from build123d import *

# Parameters (mm, degrees)
SKETCH1_W                                           = 35
SKETCH1_H                                           = 280
EXTRUDE1_DEPTH                                      = 16
EXTRUDE2_REACH                                      = 282
SKETCH2_W                                           = 15.5
SKETCH2_H                                           = 2.5
M4_TAPPED_HOLE1_D                                   = 3.3
M6_TAPPED_HOLE1_D                                   = 5
CBORE_FOR_M6_HEX_SOCKET_HEAD_CAP_SCREW1_D           = 6.6
CBORE_FOR_M6_HEX_SOCKET_HEAD_CAP_SCREW1_DEPTH       = 29
CBORE_FOR_M6_HEX_SOCKET_HEAD_CAP_SCREW1_CBORE_D     = 11
CBORE_FOR_M6_HEX_SOCKET_HEAD_CAP_SCREW1_CBORE_DEPTH = 6.4
CBORE_FOR_M6_HEX_SOCKET_HEAD_CAP_SCREW1_TIP         = 1.982840043


with BuildPart() as part:
    # Sketch1 → Extrude1 (new body)
    with BuildSketch(Plane.XY):
        Rectangle(SKETCH1_W, SKETCH1_H)
    extrude(amount=EXTRUDE1_DEPTH)

    # Sketch2 → Extrude2 (cut, up to next)
    with BuildSketch(Plane.XZ.offset(140), mode=Mode.PRIVATE) as extrude2_sk1:
        with Locations((-9.75, 14.75)):
            Rectangle(SKETCH2_W, SKETCH2_H)
    extrude2_tool1 = extrude(extrude2_sk1.sketch, amount=-EXTRUDE2_REACH, mode=Mode.PRIVATE) & part.part
    add(extrude2_tool1.solids().sort_by_distance((-9.75, -140, 14.75))[0], mode=Mode.SUBTRACT)

    # M4 Tapped Hole1 (through all)
    with Locations(Plane.XY.offset(13.5)):
        with Locations((-9.5, -120), (-9.5, -60), (-9.5, 0), (-9.5, 60), (-9.5, 120)):
            Hole(M4_TAPPED_HOLE1_D / 2)

    # M6 Tapped Hole1 (through all)
    with Locations(Plane(origin=(0, -140, 0), x_dir=(-1, 0, 0), z_dir=(0, -1, 0))):
        with Locations((-5.5, -7)):
            Hole(M6_TAPPED_HOLE1_D / 2)

    # CBORE for M6 Hex Socket Head Cap Screw1
    with Locations(Plane.XY.offset(16)):
        with Locations((0, 125), (0, 70), (0, 0), (0, -70), (0, -125)):
            CounterBoreHole(CBORE_FOR_M6_HEX_SOCKET_HEAD_CAP_SCREW1_D / 2, CBORE_FOR_M6_HEX_SOCKET_HEAD_CAP_SCREW1_CBORE_D / 2, CBORE_FOR_M6_HEX_SOCKET_HEAD_CAP_SCREW1_CBORE_DEPTH, depth=CBORE_FOR_M6_HEX_SOCKET_HEAD_CAP_SCREW1_DEPTH)
            with Locations((0, 0, -(CBORE_FOR_M6_HEX_SOCKET_HEAD_CAP_SCREW1_DEPTH + CBORE_FOR_M6_HEX_SOCKET_HEAD_CAP_SCREW1_TIP / 2))):  # 118° drill point
                Cone(0, CBORE_FOR_M6_HEX_SOCKET_HEAD_CAP_SCREW1_D / 2, CBORE_FOR_M6_HEX_SOCKET_HEAD_CAP_SCREW1_TIP, mode=Mode.SUBTRACT)


solid = part.part
Check sheet for the modelled part. Datum: model origin and axes. Units: mm. A direction names the side the tool comes from. Round coordinates to 2 decimals unless told otherwise and drop trailing zeros. Order: outer loops, then holes, each group sorted by start corner. A loop starts at its lowest first (then second) coordinate and runs counter-clockwise, first axis right, second up.
(1) Cross-section at C-C, the plane x = 0.5. State how many separate pieces and enclosed holes the cut face has, and give its area (3 significant figures).
(2) Draft check along Y on faces 1 (the flat face through (0, -140, 8)), 2 (the flat face through (0, 140, 8)), 3 (the cylindrical face through (5.246, -123.348, 12.845)), 4 (the flat face through (8, 2, 16)). Enter one of: pulls with the +Y half, pulls with the -Y half, needs draft (parallel to the pull), parting line crosses it, or undercut.
(3) Go/stop test with flat-tipped pins: P1, Ø1.2, axis at y = 134.5, z = 14.5, coming from the -X side; P2, Ø8, axis at x = -10, y = -48, coming from the +Z side; P3, Ø7.5, axis at x = 0, y = 70, coming from the +Z side. Record where each tip stops, or that it passes through.
(4) Cross-section at A-A, the plane y = 86. Enter the section's corners in (x, z), and give its area (3 significant figures).
(5) Access from +Z, -Z, +X, -X, +Y, -Y to the whole of each face (thin tool, end or side, straight path). Record for faces 5 (the flat face through (4, 0, 9.6)), 6 (the flat face through (-10, -2, 13.5)), 7 (the cylindrical face through (-3.15, -69.01, 4.73)).
(6) Scan lines: probe 1 along Y at (x, z) = (0, 2); probe 2 along Y at (x, z) = (2, 14.25); probe 3 along Z at (x, y) = (5, 68.5). Record each from-to range of solid material in increasing order.
(7) Cross-section at B-B, the plane y = -125. Enter the section's corners in (x, z), and give its area (3 significant figures).
Check sheet entries:
1. separate pieces: 6
1. enclosed holes: 0
1. area: 3,820 mm2
2. face 1: pulls with the -Y half
2. face 2: pulls with the +Y half
2. face 3: undercut
2. face 4: needs draft
3. P1: stops at x = -2
3. P2: stops at z = 13.5
3. P3: stops at z = 9.6
4. outline: (-17.5, 0) - (17.5, 0) - (17.5, 16) - (-2, 16) - (-2, 13.5) - (-17.5, 13.5) - close; hole circle Ø5 at (5.5, 7)
4. area: 502 mm2
5. face 5: +Z
5. face 6: +Z, -X, +Y, -Y
5. face 7: +Z, -Z
6. probe 1: y = -140 to -128.3, -121.7 to -73.3, -66.7 to -3.3, 3.3 to 66.7, 73.3 to 121.7, 128.3 to 140
6. probe 2: y = -140 to -130.12, -119.88 to -75.12, -64.88 to -5.12, 5.12 to 64.88, 75.12 to 119.88, 130.12 to 140
6. probe 3: z = 0 to 4.55, 9.45 to 9.6
7. outline: (-17.5, 0) - (-3.3, 0) - (-3.3, 9.6) - (-5.5, 9.6) - (-5.5, 13.5) - (-17.5, 13.5) - close; (3.3, 0) - (17.5, 0) - (17.5, 16) - (5.5, 16) - (5.5, 9.6) - (3.3, 9.6) - (3.3, 8.19) arc R2.5 cw (long way) to (3.3, 5.81) - close
7. area: 377 mm2
